from build123d import *

# Parameters (mm, degrees)
F1_DEPTH = 2438.4


with BuildPart() as f1:
    # F0 (on Front) → F1 (new body)
    with BuildSketch(Plane.XZ):
        with BuildLine():
            Line((-71.775456, 0), (106.024544, 0))
            Line((106.024544, 0), (106.024544, 53.086))
            Line((106.024544, 53.086), (103.492655, 53.086))
            ThreePointArc((103.492655, 53.086), (101.356152, 52.30165), (100.234651, 50.321224))
            Line((100.234651, 50.321224), (93.903676, 11.926927))
            ThreePointArc((93.903676, 11.926927), (91.229326, 7.204374), (86.134588, 5.334))
            Line((86.134588, 5.334), (-51.885499, 5.334))
            ThreePointArc((-51.885499, 5.334), (-56.980237, 7.204374), (-59.654587, 11.926927))
            Line((-59.654587, 11.926927), (-65.985562, 50.321224))
            ThreePointArc((-65.985562, 50.321224), (-67.107063, 52.30165), (-69.243566, 53.086))
            Line((-69.243566, 53.086), (-71.775456, 53.086))
            Line((-71.775456, 53.086), (-71.775456, 0))
        make_face()
    extrude(amount=F1_DEPTH)


solid = f1.part
Could you check a few things on this model? Use its own coordinates, in mm. A direction names the side the tool comes from. Coordinates: 2 decimals unless noted, no trailing zeros. Loops run counter-clockwise (first coordinate to the right, second up) from the corner with the lowest first, then second, coordinate; pieces in that order, holes last.
1. For P1, Ø5, axis at x = -44, y = -2033, coming from the +Z side, with a flat end and sliding along its axis, tell me the tip position at first contact or that it passes through.
2. Imagine slicing it at B-B (z = 28.5). Please give me the cut outline in (x, y), and give its area (3 significant figures).
3. Imagine slicing it at A-A (y = -1547.5). Please give me the cut outline in (x, z).
4. Imagine slicing it at C-C (x = 28). Please give me the cut outline in (y, z).
5. I need wall thicknesses on L1, parallel to X at y = -185, z = 13; L2, parallel to X at y = -841.5, z = 8.5; L3, parallel to Z at x = 30, y = -971.5. Which ranges of each line are inside material? Lowest first, please.
6. For faces 4 (the face through (18, -1202, 5.334)), 5 (the face through (106.025, -1202, 26)), which set-ups out of +Z, -Z, +X, -X, +Y, -Y let a thin tool reach every point of the face, with its end or its side?
7. We'd pull the mould along X, two halves only. Please class faces 1 (the face through (-71.775, -1202, 27)), 2 (the face through (16, -1202, 0)), 3 (the face through (97.113, -1202.131, 31.393)): released by +X, released by -X, zero draft, split by the parting line, or undercut.
Computed values:
1. P1: stops at z = 5.33
2. outline: (-71.78, -2438.4) - (-62.39, -2438.4) - (-62.39, 0) - (-71.78, 0) - close; (96.64, -2438.4) - (106.02, -2438.4) - (106.02, 0) - (96.64, 0) - close
2. area: 45,800 mm2
3. outline: (-71.78, 0) - (106.02, 0) - (106.02, 53.09) - (103.49, 53.09) arc R3.3 ccw to (100.23, 50.32) - (93.9, 11.93) arc R7.87 cw to (86.13, 5.33) - (-51.89, 5.33) arc R7.87 cw to (-59.65, 11.93) - (-65.99, 50.32) arc R3.3 ccw to (-69.24, 53.09) - (-71.78, 53.09) - close
4. outline: (-2438.4, 0) - (0, 0) - (0, 5.33) - (-2438.4, 5.33) - close
5. L1: x = -71.78 to -59.83, 94.08 to 106.02
5. L2: x = -71.78 to -58.2, 92.45 to 106.02
5. L3: z = 0 to 5.33
6. face 4: +Z, +Y, -Y
6. face 5: +Z, -Z, +X, +Y, -Y
7. face 1: released by -X
7. face 2: zero draft
7. face 3: undercut
